CAD build for the part. Positions are in the model's coordinates, mm. Face numbers are marked on the shaded views. A direction names the side the tool comes from. Give positions to 0.01 mm unless a question says otherwise; leave off trailing zeros. Loops run counter-clockwise (first coordinate to the right, second up) from the corner with the lowest first, then second, coordinate; pieces in that order, holes last.
Item 1: Saw through at A-A on y = 0. Give the cut face in (x, z), plus the area to 3 significant figures.
Item 2: Saw through at D-D on z = 1.5. Give the cut face in (x, y), plus the area to 3 significant figures.
Item 3: Saw through at B-B on x = 0. Give the cut face in (y, z).
Item 4: Probe probe 1 along Z at (x, y) = (-8.5, -3); probe 2 along Z at (x, y) = (1.5, 2.5); probe 3 along X at (y, z) = (0.5, -40.5). List the from-to ranges inside material, lowest first.
Item 5: Saw through at C-C on z = 16. Give the cut face in (x, y).
Item 6: Drop flat-ended pins along their axis: P1, Ø8, axis at y = -0.5, z = 14.5, coming from the -X side; P2, Ø1, axis at y = -2, z = -32.5, coming from the -X side; P3, Ø4, axis at y = -7.5, z = -14, coming from the -X side (3 decimals). Give the stop position or say it passes through.
Item 7: Which spindle directions (+Z, -Z, +X, -X, +Y, -Y) get a long thin tool onto all of the face, cutting with end or side? Do the marked faces 1 and 2. Say none if no direction does.
from build123d import *

# Parameters (mm, degrees)
ESQUISSE1_R             = 12.5
BOSS_EXTRU_1_DEPTH      = 65
ESQUISSE2_R             = 3.5
BOSS_EXTRU_2_DEPTH      = 2.5
ESQUISSE3_R             = 2
BOSS_EXTRU_3_DEPTH      = 22.5
ENL_V_START             = -13
ENL_V_MAT_EXTRU_1_DEPTH = 13


with BuildPart() as part:
    # Esquisse1 → Boss.-Extru.1 (new body)
    with BuildSketch(Plane.XY):
        Circle(ESQUISSE1_R)
    extrude(amount=-BOSS_EXTRU_1_DEPTH)

    # Esquisse2 → Boss.-Extru.2 (add)
    with BuildSketch(Plane.XY):
        Circle(ESQUISSE2_R)
    extrude(amount=BOSS_EXTRU_2_DEPTH)

    # Esquisse3 → Boss.-Extru.3 (add)
    with BuildSketch(Plane.XY.offset(2.5)):
        with Locations(Location((0, 0, 0), (0, 0, 180))):
            Circle(ESQUISSE3_R)
    extrude(amount=BOSS_EXTRU_3_DEPTH)

    # Esquisse4 → Enl_v. mat.-Extru.1 (cut)
    with BuildSketch(Plane.XY.offset(25).offset(ENL_V_START)):
        with BuildLine():
            Line((-1.732050808, -1), (1.732050808, -1))
            ThreePointArc((1.732050808, -1), (0, -2), (-1.732050808, -1))
        make_face()
    extrude(amount=ENL_V_MAT_EXTRU_1_DEPTH, mode=Mode.SUBTRACT)


solid = part.part
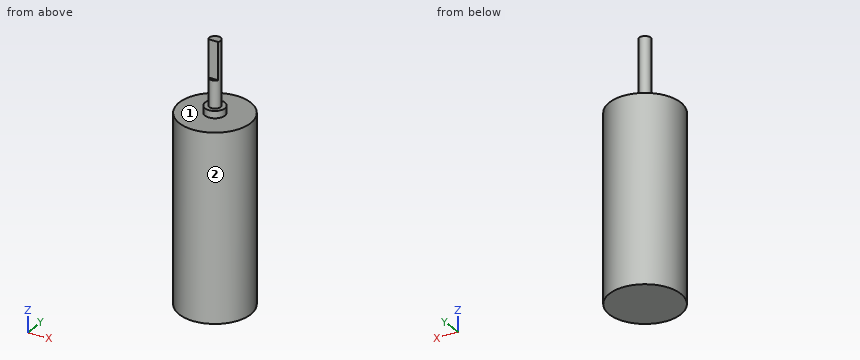
Results below:
1. outline: (-12.5, -65) - (12.5, -65) - (12.5, 0) - (3.5, 0) - (3.5, 2.5) - (2, 2.5) - (2, 25) - (-2, 25) - (-2, 2.5) - (-3.5, 2.5) - (-3.5, 0) - (-12.5, 0) - close
1. area: 1,730 mm2
2. outline: circle Ø7 at (0, 0)
2. area: 38.5 mm2
3. outline: (-12.5, -65) - (12.5, -65) - (12.5, 0) - (3.5, 0) - (3.5, 2.5) - (2, 2.5) - (2, 25) - (-1, 25) - (-1, 12) - (-2, 12) - (-2, 2.5) - (-3.5, 2.5) - (-3.5, 0) - (-12.5, 0) - close
4. probe 1: z = -65 to 0
4. probe 2: z = -65 to 2.5
4. probe 3: x = -12.49 to 12.49
5. outline: (-1.73, -1) - (1.73, -1) arc R2 ccw (long way) to start
6. P1: stops at x = -2
6. P2: stops at x = -12.41
6. P3: stops at x = -11.225
7. face 1: +Z
7. face 2: +Z, -Z
